Read the model definition and answer for the solid it produces. Units are mm, in the model's axes. A direction names the side the tool comes from. Round coordinates to 2 decimals unless told otherwise and drop trailing zeros. Write each loop counter-clockwise with the first axis right and the second up, starting at its lowest first coordinate (ties: lowest second). Pieces come first, ordered by that corner, then holes. Notation, with made-up numbers: (-10, 72) - (37, 72) arc R37 ccw to (37, 109) - close; hole circle Ø11 at (34.5, 2). An arc over 180 degrees is marked (long way). One line per item, written item: value. Start each with the question number.
(1) Flat-ended cylindrical pins translate along their axes: pin 1 Ø4.5 at (x, y) = (-84.5, 6) entering from -Z; pin 2 Ø3 at (y, z) = (7, 10.5) entering from -X; pin 3 Ø3 at (x, y) = (55.5, 3) entering from -Z. Find the tip coordinate at first contact, or state that the pin passes through.
(2) A cutting plane is placed at B-B, the plane x = 56.5. Determine the outline of the cut face in (y, z).
(3) A cutting plane is placed at C-C, the plane z = -48. Determine the outline of the cut face in (x, y), plus the area to 3 significant figures.
(4) Find the intervals of material crossed by L1, parallel to Z at x = 54, y = 12; L2, parallel to Z at x = 31.5, y = 6.25; L3, parallel to Z at x = -82.5, y = 3, in increasing order.
(5) A cutting plane is placed at A-A, the plane z = 43.5. Determine the outline of the cut face in (x, y).
(6) The mould has two halves that part along X. Classify faces 1 (the face through (-19.37, 6.26, 46.41)), 2 (the face through (28.601, 6.261, 59.963)), 3 (the face through (36, 6, 55.989)): +X half, -X half, draft (parallel to the pull), parting line (faces both ways), or undercut.
(7) For faces 4 (the face through (72.626, 6.261, 49.511)), 5 (the face through (-44.553, 6.261, 49.779)), 6 (the face through (-64.76, 6.26, -27.59)), determine the directions among +Z, -Z, +X, -X, +Y, -Y from which every point of the face is accessible in a straight line to the end or side of a thin tool.
from build123d import *

# Parameters (mm, degrees)
BOSS_EXTRUDE1_DEPTH = 12.7


with BuildPart() as part:
    # Sketch1 → Boss-Extrude1 (new body)
    with BuildSketch(Plane(origin=(0, 0, 0), x_dir=(1, 0, 0), z_dir=(0, 1, 0))):
        Polygon((-30.787184834, 46.060147433), (67.424215816, 46.060147433), (81.144259733, 46.060147433), (63.504203269, 36.260116064), (72.324231501, 30.380097243), (67.914217385, 28.322090655), (74.284237775, 14.672046963), (74.284237775, 9.604030741), (74.284237775, -4.116013175), (77.864468212, -11.787935542), (67.914217385, -16.431385928), (72.889342799, -19.748136204), (67.914217385, -27.210824325), (88.124897461, -29.905172646), (70.401780092, -47.236151197), (74.914322429, -51.850796426), (44.070310984, -51.850796426), (39.838958686, -55.98852651), (31.251122176, -55.98852651), (25.875987108, -64.051229112), (18.318515491, -59.012914701), (14.969602654, -62.287730036), (4.763594942, -51.850796426), (0, -46.979418158), (-4.105003947, -50.993595454), (-14.998499331, -39.853618754), (-23.862315978, -53.149343726), (-30.787184834, -53.149343726), (-42.728136767, -46.50148124), (-46.429188064, -53.149343726), (-52.566568213, -49.057756959), (-62.328199505, -49.057756959), (-71.736229619, -49.057756959), (-69.955147384, -35.697612338), (-64.297288709, -27.210824325), (-87.431621883, -11.787935542), (-87.431621883, -7.951974358), (-93.185563658, -4.116013175), (-88.976419646, 0), (-79.572998188, 0), (-75.864455296, 3.626488274), (-84.274708917, 12.227036224), (-78.094687193, 21.497068809), (-73.544672629, 28.322090655), (-67.126218046, 24.043120934), (-62.328199505, 31.240148746), (-68.47808372, 44.418472064), (-59.570897098, 57.779251997), align=None)
        with BuildLine():
            Line((-11.923576625, 7.986340539), (-8.84865392, 3.609452157))
            Line((-8.84865392, 3.609452157), (-19.546747498, 3.609452157))
            ThreePointArc((-19.546747498, 3.609452157), (-23.034496934, 4.839852529), (-24.978177568, 7.986340539))
            Line((-24.978177568, 7.986340539), (-27.332016626, 12.363228921))
            Line((-27.332016626, 12.363228921), (-21.358576046, 14.422806945))
            ThreePointArc((-21.358576046, 14.422806945), (-17.834303779, 14.456028923), (-14.998499331, 12.363228921))
            Line((-14.998499331, 12.363228921), (-8.84865392, 12.363228921))
            Line((-8.84865392, 12.363228921), (-11.923576625, 7.986340539))
        make_face(mode=Mode.SUBTRACT)
    extrude(amount=BOSS_EXTRUDE1_DEPTH)


solid = part.part
Here are the results:
1. pin 1: z = -15.26
1. pin 2: x = -87.43
1. pin 3: z = -46.06
2. outline: (0, -46.06) - (12.7, -46.06) - (12.7, 51.85) - (0, 51.85) - close
3. outline: (-66.09, 0) - (-35.55, 0) - (-35.55, 12.7) - (-66.09, 12.7) - close
3. area: 388 mm²
4. L1: -46.06 to 51.85
4. L2: -46.06 to 55.99
4. L3: -14.89 to -10.41, 0 to 15.08
5. outline: (-71, 0) - (-17.43, 0) - (-17.43, 12.7) - (-71, 12.7) - close; (-11.43, 0) - (74.22, 0) - (74.22, 12.7) - (-11.43, 12.7) - close
6. face 1: undercut
6. face 2: +X half
6. face 3: draft
7. face 4: +X, +Y, -Y
7. face 5: +Z, +Y, -Y
7. face 6: +Y, -Y
